Read the model definition and answer for the solid it produces. Units are mm, in the model's axes. A direction names the side the tool comes from. Coordinates: 2 decimals unless noted, no trailing zeros. Order: outer loops, then holes, each group sorted by start corner. A loop starts at its lowest first (then second) coordinate and runs counter-clockwise, first axis right, second up. Notation, with made-up numbers: (48.25, 22.5) - (84.25, 22.5) arc R20 cw to (84.25, 29.5) - close; hole circle Ø1 at (55.5, 75.5). An arc over 180 degrees is marked (long way). Answer as a JSON object with one key per item and string values. Group by question number.
from build123d import *

# Parameters (mm, degrees)
SKETCH1_R           = 20
BOSS_EXTRUDE4_DEPTH = 40
BOSS_EXTRUDE5_START = 5
BOSS_EXTRUDE5_DEPTH = 5
SKETCH6_R           = 1.25
CUT_EXTRUDE1_DEPTH  = 5
SKETCH7_R           = 3
CUT_EXTRUDE2_DEPTH  = 2
SKETCH8_R           = 20.25
CUT_EXTRUDE3_DEPTH  = 40
SKETCH9_W           = 42.5
SKETCH9_H           = 42.5
CUT_EXTRUDE4_DEPTH  = 40
SKETCH10_W          = 18.5
SKETCH10_H          = 40
CUT_EXTRUDE5_DEPTH  = 7
SKETCH11_R          = 1.6
CUT_EXTRUDE6_DEPTH  = 269.248997311


with BuildPart() as part:
    # Sketch1 → Boss-Extrude4 (new body)
    with BuildSketch(Plane(origin=(0, 0, 0), x_dir=(0, 1, 0), z_dir=(0, 0, 1))):
        with BuildLine():
            Line((48.86109499, -159.669791534), (48.86109499, -209.83599005))
            Line((48.86109499, -209.83599005), (65.86109499, -209.83599005))
            Line((65.86109499, -209.83599005), (65.86109499, -204.83599005))
            Line((65.86109499, -204.83599005), (53.86109499, -204.83599005))
            Line((53.86109499, -204.83599005), (53.86109499, -163.588668859))
            Line((53.86109499, -163.588668859), (95.86109499, -163.588668859))
            Line((95.86109499, -163.588668859), (95.86109499, -204.83599005))
            Line((95.86109499, -204.83599005), (83.86109499, -204.83599005))
            Line((83.86109499, -204.83599005), (83.86109499, -209.83599005))
            Line((83.86109499, -209.83599005), (100.86109499, -209.83599005))
            Line((100.86109499, -209.83599005), (100.86109499, -159.603176712))
            ThreePointArc((100.86109499, -159.603176712), (74.64197355, 11.411259343), (48.86109499, -159.669791534))
        make_face()
        with Locations(Location((74.754065705, -76.088668859, 0), (0, 0, 270))):
            Circle(SKETCH1_R, mode=Mode.SUBTRACT)
        with BuildLine():
            Line((149.524530838, -70.225432227), (106.720805548, -70.225432227))
            ThreePointArc((106.720805548, -70.225432227), (97.065220712, -52.456860586), (78.771338454, -43.837908873))
            Line((78.771338454, -43.837908873), (78.771338454, -1.19633601))
            ThreePointArc((78.771338454, -1.19633601), (127.128973259, -22.405626297), (149.524530838, -70.225432227))
        make_face(mode=Mode.SUBTRACT)
        with BuildLine():
            Line((149.682278397, -79.369361301), (107.088057991, -79.369361301))
            ThreePointArc((107.088057991, -79.369361301), (98.250620194, -98.542219295), (79.498497507, -108.240501884))
            Line((79.498497507, -108.240501884), (79.498497507, -150.938454209))
            ThreePointArc((79.498497507, -150.938454209), (128.302794309, -128.600892817), (149.682278397, -79.369361301))
        make_face(mode=Mode.SUBTRACT)
        with BuildLine():
            Line((70.783231418, -150.983478259), (70.783231418, -108.345179443))
            ThreePointArc((70.783231418, -108.345179443), (51.584378521, -98.879359849), (42.436457903, -79.52701525))
            Line((42.436457903, -79.52701525), (-0.167078, -79.52701525))
            ThreePointArc((-0.167078, -79.52701525), (21.532899104, -128.932849482), (70.783231418, -150.983478259))
        make_face(mode=Mode.SUBTRACT)
        with BuildLine():
            Line((-0.003869503, -70.067778277), (42.816644448, -70.067778277))
            ThreePointArc((42.816644448, -70.067778277), (52.673264417, -52.241484236), (71.203948876, -43.783148116))
            Line((71.203948876, -43.783148116), (71.203948876, -1.172738174))
            ThreePointArc((71.203948876, -1.172738174), (22.603616127, -22.187550051), (-0.003869503, -70.067778277))
        make_face(mode=Mode.SUBTRACT)
    extrude(amount=BOSS_EXTRUDE4_DEPTH)

    # Sketch4 → Boss-Extrude5 (add)
    with BuildSketch(Plane(origin=(0, 0, 0), x_dir=(1, 0, 0), z_dir=(0, 0, -1)).offset(BOSS_EXTRUDE5_START)):
        with BuildLine():
            Line((159.669791534, -48.86109499), (209.83599005, -48.86109499))
            Line((209.83599005, -48.86109499), (209.83599005, -100.86109499))
            Line((209.83599005, -100.86109499), (159.603176712, -100.86109499))
            ThreePointArc((159.603176712, -100.86109499), (-11.411259343, -74.64197355), (159.669791534, -48.86109499))
        make_face()
    extrude(amount=-BOSS_EXTRUDE5_DEPTH)

    # Sketch6 → Cut-Extrude1 (cut)
    with BuildSketch(Plane(origin=(0, 0, -5), x_dir=(1, 0, 0), z_dir=(0, 0, -1))):
        with Locations(Location((199.962329455, -59.61109499, 0), (0, 0, 180))):
            Circle(SKETCH6_R)
        with Locations(Location((168.962329455, -59.61109499, 0), (0, 0, 180))):
            Circle(SKETCH6_R)
        with Locations(Location((168.962329455, -90.61109499, 0), (0, 0, 180))):
            Circle(SKETCH6_R)
        with Locations(Location((199.962329455, -90.61109499, 0), (0, 0, 180))):
            Circle(SKETCH6_R)
    extrude(amount=-CUT_EXTRUDE1_DEPTH, mode=Mode.SUBTRACT)

    # Sketch7 → Cut-Extrude2 (cut)
    with BuildSketch(Plane(origin=(0, 0, -5), x_dir=(-1, 0, 0), z_dir=(0, 0, -1))):
        with Locations((-199.962329455, 59.61109499)):
            Circle(SKETCH7_R)
        with Locations((-168.962329455, 59.61109499)):
            Circle(SKETCH7_R)
        with Locations((-168.962329455, 90.61109499)):
            Circle(SKETCH7_R)
        with Locations((-199.962329455, 90.61109499)):
            Circle(SKETCH7_R)
    extrude(amount=-CUT_EXTRUDE2_DEPTH, mode=Mode.SUBTRACT)

    # Sketch8 → Cut-Extrude3 (cut)
    with BuildSketch(Plane.XY.offset(40)):
        with Locations((76.088668859, 74.754065705)):
            Circle(SKETCH8_R)
    extrude(amount=-CUT_EXTRUDE3_DEPTH, mode=Mode.SUBTRACT)

    # Sketch9 → Cut-Extrude4 (cut)
    with BuildSketch(Plane.XY.offset(40)):
        with Locations((184.212329455, 74.86109499)):
            Rectangle(SKETCH9_W, SKETCH9_H)
    extrude(amount=-CUT_EXTRUDE4_DEPTH, mode=Mode.SUBTRACT)

    # Sketch10 → Cut-Extrude5 (cut)
    with BuildSketch(Plane.YZ.offset(209.83599005)):
        with Locations((74.86109499, 20)):
            Rectangle(SKETCH10_W, SKETCH10_H)
    extrude(amount=-CUT_EXTRUDE5_DEPTH, mode=Mode.SUBTRACT)

    # Sketch11 → Cut-Extrude6 (cut, through all)
    with BuildSketch(Plane.XY):
        with Locations((168.962329455, 90.61109499)):
            Circle(SKETCH11_R)
        with Locations((199.962329455, 90.61109499)):
            Circle(SKETCH11_R)
        with Locations((168.962329455, 59.61109499)):
            Circle(SKETCH11_R)
        with Locations((199.962329455, 59.61109499)):
            Circle(SKETCH11_R)
    extrude(amount=-CUT_EXTRUDE6_DEPTH, mode=Mode.SUBTRACT)


solid = part.part
1. Straight lines are drawn through the part: L1, parallel to Y at x = 99.5, z = 9.5; L2, parallel to Y at x = 123, z = 14; L3, parallel to X at y = 13, z = 14. For each, find the intervals that lie inside material, in ascending order.
2. A cutting plane is placed at B-B on x = 13.5. Write down the section's boundary in (y, z).
3. A cutting plane is placed at A-A on z = 5. State how many separate pieces and enclosed holes the cut face has, and give its area (3 significant figures).
4. Given pin 1 (8 mm diameter, centred on x = 128.5, y = 114.5, fed in from +Z); pin 2 (22.5 mm diameter, centred on x = 183, z = 24, fed in from -Y); pin 3 (8 mm diameter, centred on x = 173.5, z = 21.5, fed in from +Y), each flat-ended and moving along its own axis, determine where each tip first touches the part or whether it passes through.
5. A cutting plane is placed at C-C on y = 130.5. Write down the section's boundary in (x, z).
6. For faces 3 (the flat face through (208, 65.611, 20)), 4 (the flat face through (116, 114, 0)), 5 (the flat face through (199, 58, -3)), determine the directions among +Z, -Z, +X, -X, +Y, -Y from which every point of the face is accessible in a straight line to the end or side of a thin tool.
7. For a pull along Y with two mould halves and no side action, classify faces 1 (the cylindrical face through (-11.347, 78.12, 17.185)), 2 (the cylindrical face through (171.17, 61.64, -4.01)) as pulls with the +Y half, pulls with the -Y half, needs draft (parallel to the pull), parting line crosses it, or undercut.
Derived:
{
 "1": {"L1": "y = -9.56 to 3.5, 52.21 to 97.3, 146.01 to 159.06", "L2": "y = 0.89 to 16.24, 70.78 to 79.5, 133.27 to 148.62", "L3": "x = 14.1 to 33.53, 70.07 to 79.53, 118.65 to 138.08"},
 "2": {"outline": "(13.61, -5) - (135.9, -5) - (135.9, 40) - (116.08, 40) - (116.08, 0) - (78.77, 0) - (78.77, 40) - (71.2, 40) - (71.2, 0) - (33.43, 0) - (33.43, 40) - (13.61, 40) - close"},
 "3": {"separate pieces": "1", "enclosed holes": "5", "area": "10,500 mm2"},
 "4": {"pin 1": "stops at z = 0", "pin 2": "stops at y = 48.86", "pin 3": "stops at y = 100.86"},
 "5": {"outline": "(8.65, -5) - (143.53, -5) - (143.53, 40) - (126.26, 40) - (126.26, 0) - (79.37, 0) - (79.37, 40) - (70.23, 40) - (70.23, 0) - (25.92, 0) - (25.92, 40) - (8.65, 40) - close"},
 "6": {"face 3": "+Z, +X", "face 4": "+Z", "face 5": "-Z"},
 "7": {"face 1": "parting line crosses it", "face 2": "undercut"}
}
